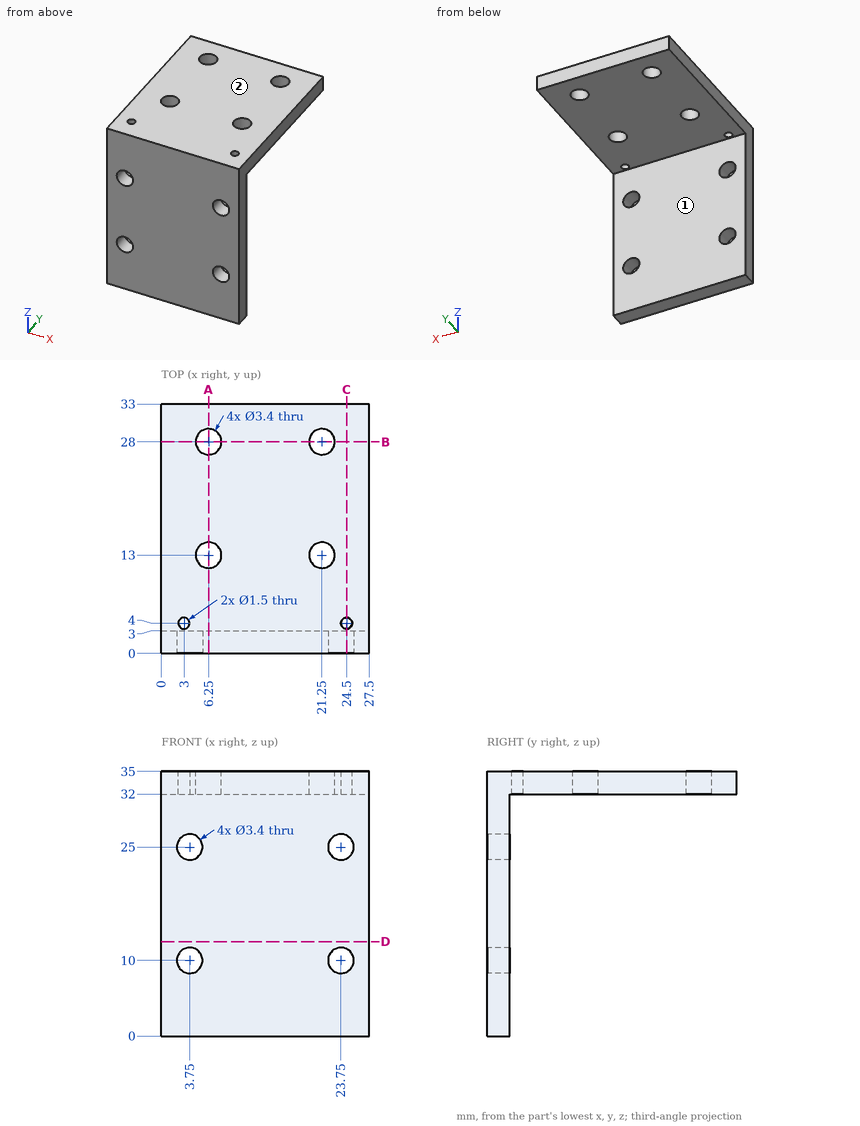
The drawing under review shows one solid part. Ordinate dimensions are in mm from its lowest x, y, z. A direction names the side the tool comes from. Round coordinates to 2 decimals unless told otherwise and drop trailing zeros. Order: outer loops, then holes, each group sorted by start corner. A loop starts at its lowest first (then second) coordinate and runs counter-clockwise, first axis right, second up. Notation, with made-up numbers: (74.25, 16) -> (131.25, 16) arc R14 ccw to (131.25, 35) -> close; hole circle Ø3 at (-3, -35.75). An arc over 180 degrees is marked (long way). Return JSON: item names as keys, results as strings.
1. Take a section at B-B (y = 28). Write out the cut boundary in (x, z), then the cut area to 3 significant figures.
Answer block:
{"outline": "(0, 32) -> (4.55, 32) -> (4.55, 35) -> (0, 35) -> close; (7.95, 32) -> (19.55, 32) -> (19.55, 35) -> (7.95, 35) -> close; (22.95, 32) -> (27.5, 32) -> (27.5, 35) -> (22.95, 35) -> close", "area": "62.1 mm²"}
2. Take a section at A-A (x = 6.25). Write out the cut boundary in (y, z).
Answer block:
{"outline": "(0, 0) -> (3, 0) -> (3, 32) -> (11.3, 32) -> (11.3, 35) -> (0, 35) -> close; (14.7, 32) -> (26.3, 32) -> (26.3, 35) -> (14.7, 35) -> close; (29.7, 32) -> (33, 32) -> (33, 35) -> (29.7, 35) -> close"}
3. Take a section at D-D (z = 12.5). Write out the cut boundary in (x, y).
Answer block:
{"outline": "(0, 0) -> (27.5, 0) -> (27.5, 3) -> (0, 3) -> close"}
4. Insertion check: P1, Ø4, axis at x = 6.25, y = 13, coming from the -Z side; P2, Ø8, axis at x = 23, z = 17.5, coming from the -Y side; P3, Ø6, axis at x = 10, z = 16, coming from the +Y side. Each pin has a flat end and moves straight along its axis. Give the tip position at first contact, or say it passes through.
Answer block:
{"P1": "stops at z = 32", "P2": "stops at y = 0", "P3": "stops at y = 3"}
5. For L1, parallel to Z at x = 3.75, y = 0.75; L2, parallel to X at y = 2.15, z = 10; L3, parallel to Y at x = 21.25, z = 33.7, list the stretches that pass through material, from the lowest coordinate up. Write a range as [from, to].
Answer block:
{"L1": "z = [0, 8.3], [11.7, 23.3], [26.7, 35]", "L2": "x = [0, 2.05], [5.45, 22.05], [25.45, 27.5]", "L3": "y = [0, 11.3], [14.7, 26.3], [29.7, 33]"}
6. For the marked faces 1 and 2, list the 3-axis set-ups (+Z, -Z, +X, -X, +Y, -Y) from which the entire face can be reached by the end or side of a thin tool; tool diameter is ignored.
Answer block:
{"face 1": "-Z, +X, -X, +Y", "face 2": "+Z, +X, -X, +Y, -Y"}
7. Take a section at C-C (x = 24.5). Write out the cut boundary in (y, z).
Answer block:
{"outline": "(0, 0) -> (3, 0) -> (3, 8.47) -> (0, 8.47) -> close; (0, 11.53) -> (3, 11.53) -> (3, 23.47) -> (0, 23.47) -> close; (0, 26.53) -> (3, 26.53) -> (3, 32) -> (3.25, 32) -> (3.25, 35) -> (0, 35) -> close; (4.75, 32) -> (33, 32) -> (33, 35) -> (4.75, 35) -> close"}
